Geometry: final body of the model. Coordinates: model frame, mm. A direction names the side the tool comes from. Coordinates: 2 decimals unless noted, no trailing zeros. Write each loop counter-clockwise with the first axis right and the second up, starting at its lowest first coordinate (ties: lowest second). Pieces come first, ordered by that corner, then holes.
from build123d import *

# Parameters (mm, degrees)
SKETCH_1_R               = 25
SKETCH_1_R_2             = 1.525
EXTRUDE_1_DEPTH          = 3
EXTRUDE_START            = -3
SKETCH_2_R               = 4
EXTRUDE_2_DEPTH          = 11.3
SKETCH_3_R               = 5.2
EXTRUDE_3_DEPTH          = 1.2
HOLE_WIZARD_M4_1_D       = 3.3
SKETCH_6_W               = 9
SKETCH_6_H               = 2.1
CUT_EXTRUDE_1_DEPTH      = 26
CUT_EXTRUDE_1_DEPTH_BACK = 26


with BuildPart() as part:
    # 草图1 → 凸台-拉伸1 (new body)
    with BuildSketch(Plane.XY):
        Circle(SKETCH_1_R)
        with Locations((0, 19)):
            Circle(SKETCH_1_R_2, mode=Mode.SUBTRACT)
        with Locations((13.435028843, 13.435028843)):
            Circle(SKETCH_1_R_2, mode=Mode.SUBTRACT)
        with Locations((19, 0)):
            Circle(SKETCH_1_R_2, mode=Mode.SUBTRACT)
        with Locations((13.435028843, -13.435028843)):
            Circle(SKETCH_1_R_2, mode=Mode.SUBTRACT)
        with Locations((0, -19)):
            Circle(SKETCH_1_R_2, mode=Mode.SUBTRACT)
        with Locations((-13.435028843, -13.435028843)):
            Circle(SKETCH_1_R_2, mode=Mode.SUBTRACT)
        with Locations((-19, 0)):
            Circle(SKETCH_1_R_2, mode=Mode.SUBTRACT)
        with Locations((-13.435028843, 13.435028843)):
            Circle(SKETCH_1_R_2, mode=Mode.SUBTRACT)
    extrude(amount=EXTRUDE_1_DEPTH)

    # 草图2 → 凸台-拉伸2 (add)
    with BuildSketch(Plane.XY.offset(3).offset(EXTRUDE_START)):
        Circle(SKETCH_2_R)
    extrude(amount=-EXTRUDE_2_DEPTH)

    # 草图3 → 凸台-拉伸3 (add)
    with BuildSketch(Plane.XY.offset(3).offset(EXTRUDE_START)):
        Circle(SKETCH_3_R)
    extrude(amount=-EXTRUDE_3_DEPTH)

    # M4 螺纹孔1 (through all)
    with Locations(Plane(origin=(0, 0, -11.3), x_dir=(-1, 0, 0), z_dir=(0, 0, -1))):
        with Locations((0, 0)):
            Hole(HOLE_WIZARD_M4_1_D / 2)

    # 草图6 → 切除-拉伸1 (cut, two sides)
    with BuildSketch(Plane(origin=(0, 0, 0), x_dir=(1, 0, 0), z_dir=(0, 1, 0))) as cut_extrude_1_sk:
        with Locations((-0.5, 10.25)):
            Rectangle(SKETCH_6_W, SKETCH_6_H)
    extrude(amount=CUT_EXTRUDE_1_DEPTH, mode=Mode.SUBTRACT)
    extrude(cut_extrude_1_sk.sketch, amount=-CUT_EXTRUDE_1_DEPTH_BACK, mode=Mode.SUBTRACT)


solid = part.part
Item 1: Material intervals for probe 1 along Y at (x, z) = (0, 1.15) (3 decimals); probe 2 along Y at (x, z) = (0, -5.75); probe 3 along Z at (x, y) = (-13, -18), sorted ascending.
Derived:
probe 1: y = -25 to -20.525, -17.475 to -1.65, 1.65 to 17.475, 20.525 to 25
probe 2: y = -4 to -1.65, 1.65 to 4
probe 3: z = 0 to 3
Item 2: Section B-B, the plane y = 19. Output: boundary loops of the cut face in (x, z) (3 decimals), plus the area to 3 significant figures.
Derived:
outline: (-16.248, 0) - (-1.525, 0) - (-1.525, 3) - (-16.248, 3) - close; (1.525, 0) - (16.248, 0) - (16.248, 3) - (1.525, 3) - close
area: 88.3 mm2
Item 3: Section A-A, the plane x = 0. Output: boundary loops of the cut face in (y, z) (3 decimals), plus the area to 3 significant figures.
Derived:
outline: (-25, 0) - (-20.525, 0) - (-20.525, 3) - (-25, 3) - close; (-17.475, 0) - (-5.2, 0) - (-5.2, -1.2) - (-4, -1.2) - (-4, -9.2) - (-1.65, -9.2) - (-1.65, 3) - (-17.475, 3) - close; (1.65, -9.2) - (4, -9.2) - (4, -1.2) - (5.2, -1.2) - (5.2, 0) - (17.475, 0) - (17.475, 3) - (1.65, 3) - close; (20.525, 0) - (25, 0) - (25, 3) - (20.525, 3) - close
area: 168 mm2
Item 4: Section C-C, the plane x = -13. Output: boundary loops of the cut face in (y, z), plus the area to 3 significant figures.
Derived:
outline: (-21.35, 0) - (-14.9, 0) - (-14.9, 3) - (-21.35, 3) - close; (-11.97, 0) - (11.97, 0) - (11.97, 3) - (-11.97, 3) - close; (14.9, 0) - (21.35, 0) - (21.35, 3) - (14.9, 3) - close
area: 111 mm2
Item 5: Pull-direction query (X, two-part tool) for faces 3 (the cylindrical face through (14.255, -12.149, 1.479)), 4 (the cylindrical face through (-0.867, -3.905, -5.144)), 5 (the flat face through (0, 6, 0)); classes: released by +X, released by -X, zero draft, split by the parting line, or undercut.
Derived:
face 3: undercut
face 4: split by the parting line
face 5: zero draft
Item 6: Section D-D, the plane z = -7.25. Output: boundary loops of the cut face in (x, y).
Derived:
outline: circle Ø8 at (0, 0); hole circle Ø3.3 at (0, 0)
Item 7: Set-up query: faces 1 (the cylindrical face through (-0.677, 5.156, -0.592)), 2 (the cylindrical face through (-14.96, 13.5, 1.48)). Return all of +Z, -Z, +X, -X, +Y, -Y with unobstructed straight access to the full face (end or side cutting, diameter ignored); none if empty.
Derived:
face 1: -Z
face 2: +Z, -Z
Item 8: Pin query (flat end, axial travel): pin 1 (5 mm diameter, centred on x = -19, y = 0, fed in from -Z); pin 2 (5 mm diameter, centred on y = 14, z = 0, fed in from +X); pin 3 (6 mm diameter, centred on x = -20, z = -1.5, fed in from +Y). Return the tip coordinate at first contact, or that it passes through.
Derived:
pin 1: stops at z = 0
pin 2: stops at x = 22.2
pin 3: stops at y = 17.95
